For this review, take the finished solid that the model builds, in its own axes (mm). A direction names the side the tool comes from. Round coordinates to 2 decimals unless told otherwise and drop trailing zeros. Loops run counter-clockwise (first coordinate to the right, second up) from the corner with the lowest first, then second, coordinate; pieces in that order, holes last.
1) Take a section at A-A (x = 0). State the section outline as (y, z) points.
2) Tool access review of faces 5 (the cylindrical face through (-20.03, -6.31, -0.99)), 6 (the flat face through (0, 3.5, 55)), 7 (the cylindrical face through (0.2, -12.5, 40.2)), 8 (the flat face through (12, 12, 33.2)): name each direction out of +Z, -Z, +X, -X, +Y, -Y from which nothing blocks a thin tool from reaching the whole face with its end or side.
3) Wall thickness on L1, parallel to Z at x = 2.5, y = 6.5; L2, parallel to Z at x = -8, y = 19; L3, parallel to X at y = -3.5, z = 42.5: over which ranges is each line inside the solid? List them lowest first.
4) Mouldability with a two-part tool opening along Y and no side actions: class faces 1 (the cylindrical face through (-0.2, 12.5, 40.2)), 2 (the flat face through (12, -12, 33.2)), 3 (the flat face through (9, -9, 39.2)), 4 (the cylindrical face through (10.9, 13.726, 36.242)) as pulls with the +Y half, pulls with the -Y half, needs draft (parallel to the pull), parting line crosses it, or undercut.
5) Take a section at D-D (z = 29). State the section outline as (x, y) points, then the cut area to 3 significant figures.
6) Take a section at B-B (z = -68). State the section outline as (x, y) points.
7) Insertion check: pin 1 (3 mm diameter, centred on x = 13, y = 12, fed in from +Z); pin 2 (3.5 mm diameter, centred on x = 12.37, y = 12.37, fed in from +Z); pin 3 (10 mm diameter, centred on y = -8, z = -7.5, fed in from -X); pin 4 (10 mm diameter, centred on y = 3, z = -39, fed in from +X). Each pin has a flat end and moves straight along its axis. Give the tip position at first contact, or say it passes through.
8) Take a section at C-C (x = 8.5). State the section outline as (y, z) points.
Autodesk Inventor part; units mm, degrees
ref_plane "YZ Plane" through (0, 0, 0) normal (1, 0, 0) x (0, 1, 0)
ref_plane "XZ Plane" through (0, 0, 0) normal (0, 1, 0) x (-1, 0, 0)
ref_plane "XY Plane" through (0, 0, 0) normal (0, 0, 1) x (1, 0, 0)
sketch "스케치1" plane through (0, 0, 0) normal (0, 0, 1) x (1, 0, 0)
  circle A0 centre (0, 0) radius 21.2
  dimension "d0" = 42.4
extrude "돌출1" add sketch "스케치1" along normal blind 39.2
sketch "스케치2" plane through (0, 0, 0) normal (0, 0, -1) x (-1, 0, 0)
  circle A0 centre (0, 0) radius 21
  dimension "d5" = 42
extrude "돌출2" add sketch "스케치2" along normal blind 2
sketch "스케치3" plane through (0, 0, -2) normal (0, 0, -1) x (-1, 0, 0)
  circle A0 centre (0, 0) radius 21.2
extrude "돌출3" add sketch "스케치3" along normal blind 64
sketch "스케치4" plane through (0, 0, -66) normal (0, 0, -1) x (-1, 0, 0)
  circle A0 centre (0, 0) radius 21.15
  dimension "d19" = 42.3
extrude "돌출4" add sketch "스케치4" along normal blind 15
sketch "스케치5" plane through (0, 0, 39.2) normal (0, 0, 1) x (1, 0, 0)
  circle A0 centre (0, 0) radius 12.5
  line L0 (0, 0) -> (11.5, 0)
  line L1 (11.5, 0) -> (11.5, 4.899)
  line L2 (11.5, 0) -> (11.5, -4.899)
  line L3 (0, 0) -> (-11.5, 0)
  line L4 (-11.5, 0) -> (-11.5, 4.899)
  line L5 (-11.5, 0) -> (-11.5, -4.899)
  dimension "d10" = 25
  dimension "d20" = 11.5
  dimension "d21" = 11.5
extrude "돌출5" add sketch "스케치5" along normal blind 2 contours L1 L0 L3 L4 A0 | A0 L5 L3 L0 L2
sketch "스케치6" plane through (0, 0, 41.2) normal (0, 0, 1) x (-1, 0, 0)
  circle A0 centre (0, 0) radius 4
  dimension "d13" = 8
extrude "돌출6" add sketch "스케치6" along normal blind 8
sketch "스케치7" plane through (0, 0, 49.2) normal (0, 0, 1) x (1, 0, 0)
  line L0 (0, 0) -> (0, 3.5)
  line L1 (0, 3.5) -> (1.9365, 3.5)
  circle A0 centre (0, 0) radius 4
  line L2 (0, 3.5) -> (-1.9365, 3.5)
  arc A1 (-1.9365, 3.5) -> (1.9365, 3.5) centre (0, 0) ccw
  dimension "d16" = 3.5
extrude "돌출7" add sketch "스케치7" along normal blind 12 contours L1 A0 L2 picked at (-0.0999, -1.4777)
sketch "스케치8" plane through (0, 0, 39.2) normal (0, 0, 1) x (1, 0, 0)
  arc A0 (11.5, 4.899) -> (-11.5, 4.899) centre (0, 0) ccw
  line L0 (11.5, 4.899) -> (11.5, -4.899)
  arc A1 (-11.5, -4.899) -> (11.5, -4.899) centre (0, 0) ccw
  line L1 (-11.5, -4.899) -> (-11.5, 4.899)
  circle A2 centre (0, 0) radius 21.2
  line L2 (0, 0) -> (12.3744, 12.3744)
  line L3 (0, 0) -> (17.5, 0) construction
  circle A3 centre (12.3744, 12.3744) radius 2
  circle A4 centre (-12.3744, 12.3744) radius 2
  circle A5 centre (-12.3744, -12.3744) radius 2
  circle A6 centre (12.3744, -12.3744) radius 2
  dimension "d22" = 17.5
  dimension "d23" = 45
  dimension "d24" = 4
  dimension "d27" = 360
extrude "돌출8" cut sketch "스케치8" against normal blind 6 contours A3 | A4 | A5 | A6
thread "스레드1"
thread "스레드2"
thread "스레드3"
thread "스레드4"
properties part number "IG-42GM_motor"
Response:
1. outline: (-21.2, -66) - (-21.15, -66) - (-21.15, -81) - (21.15, -81) - (21.15, -66) - (21.2, -66) - (21.2, -2) - (21, -2) - (21, 0) - (21.2, 0) - (21.2, 39.2) - (12.5, 39.2) - (12.5, 41.2) - (4, 41.2) - (4, 49.2) - (3.5, 49.2) - (3.5, 61.2) - (-4, 61.2) - (-4, 41.2) - (-12.5, 41.2) - (-12.5, 39.2) - (-21.2, 39.2) - (-21.2, 0) - (-21, 0) - (-21, -2) - (-21.2, -2) - close
2. face 5: none
2. face 6: +Z, +X, -X, +Y
2. face 7: +Z, -Y
2. face 8: +Z
3. L1: z = -81 to 41.2
3. L2: z = -81 to 39.2
3. L3: x = -1.94 to 1.94
4. face 1: pulls with the +Y half
4. face 2: undercut
4. face 3: needs draft
4. face 4: undercut
5. outline: circle Ø42.4 at (0, 0)
5. area: 1,410 mm2
6. outline: circle Ø42.3 at (0, 0)
7. pin 1: stops at z = 39.2
7. pin 2: stops at z = 33.2
7. pin 3: stops at x = -20.99
7. pin 4: stops at x = 21.2
8. outline: (-19.42, -66) - (-19.37, -66) - (-19.37, -81) - (19.37, -81) - (19.37, -66) - (19.42, -66) - (19.42, -2) - (19.2, -2) - (19.2, 0) - (19.42, 0) - (19.42, 39.2) - (9.17, 39.2) - (9.17, 41.2) - (-9.17, 41.2) - (-9.17, 39.2) - (-19.42, 39.2) - (-19.42, 0) - (-19.2, 0) - (-19.2, -2) - (-19.42, -2) - close
